```python
from build123d import *

# Parameters (mm, degrees)
F1_DEPTH = 50
F3_DEPTH = 50


with BuildPart() as f1:
    # F0 (on Front) → F1 (new body)
    with BuildSketch(Plane.XZ):
        Polygon((-34.2579181991, 25.4109162267), (-75.2579181991, 25.4109162267), (-75.2579181991, -22.5890837733), (74.7420818009, -22.5890837733), (74.7420818009, 25.4109162267), (33.7420818009, 25.4109162267), (33.7420818009, 0), (-34.2579181991, 0), align=None)
    extrude(amount=F1_DEPTH)

    # F2 (on Front) → F3 (join)
    with BuildSketch(Plane.XZ):
        with BuildLine():
            add(Edge.make_bspline(
                [(-34.439124167, 25.7045440376), (-29.8644360155, 7.841472514), (-15.2597080741, 0.0492694303), (0, 0)],
                knots=[0, 0, 0, 0, 0.5003378165, 0.5003378165, 0.5003378165, 0.5003378165], degree=3))
            Line((-34.439124167, 25.7045440376), (-34.439124167, 0))
            Line((-34.439124167, 0), (0, 0))
        make_face()
        with BuildLine():
            add(Edge.make_bspline(
                [(0.2911255263, 0), (15.4409229129, 0.0489315649), (31.1494455799, 7.7415126091), (33.9633673429, 26.1402279139)],
                knots=[0.503518811, 0.503518811, 0.503518811, 0.503518811, 1, 1, 1, 1], degree=3))
            Line((0.2911255263, 0), (33.9633673429, 0))
            Line((33.9633673429, 0), (33.9633673429, 26.1402279139))
        make_face()
        with BuildLine():
            Line((0.2911255263, 0), (0, 0))
            add(Edge.make_bspline(
                [(0, 0), (0.0970165471, -0.0003132399), (0.1940595687, -0.0003135084), (0.2911255263, 0)],
                knots=[0.5003378165, 0.5003378165, 0.5003378165, 0.5003378165, 0.503518811, 0.503518811, 0.503518811, 0.503518811], degree=3))
        make_face()
    extrude(amount=F3_DEPTH)


solid = f1.part
```
Build history of the part. All positions in model axes, mm. A direction names the side the tool comes from. Give positions to 0.01 mm unless a question says otherwise; leave off trailing zeros. Write item = value, one per line. Start each with the question number.
(1) Pin check, flat tips, straight feed: pin 1 Ø20.5 at (x, y) = (-64, -36.5) entering from +Z; pin 2 Ø12 at (x, y) = (15, -5.5) entering from +Z; pin 3 Ø8 at (x, y) = (-10, -17.5) entering from +Z. Stop position of each tip, or through.
(2) Which spindle directions (+Z, -Z, +X, -X, +Y, -Y) get a long thin tool onto all of the face, cutting with end or side? Do faces 1 (the flat face through (1, -50, -3)), 2 (the flat face through (55, -25, 25.411)), 3 (the flat face through (-55, -25, 25.411)). Say none if no direction does.
(3) Probe L1, parallel to Z at x = 40, y = -29; L2, parallel to X at y = -11.5, z = 5.5; L3, parallel to X at y = -5.5, z = 19.5. List the from-to ranges inside material, lowest first. Write a range as [from, to].
Responses:
q1.pin_1 = 25.41
q1.pin_2 = 5.69
q1.pin_3 = 2.45
q2.face_1 = +Z, -Z, +X, -X, -Y
q2.face_2 = +Z, +X, +Y, -Y
q2.face_3 = +Z, -X, +Y, -Y
q3.L1 = [-22.59, 25.41]
q3.L2 = [-75.26, -20.2], [20.7, 74.74]
q3.L3 = [-75.26, -32.28], [32.24, 74.74]
